Design review of the part built by this model. Coordinates are the model's own, in mm. A direction names the side the tool comes from. Coordinates: 2 decimals unless noted, no trailing zeros. Loops run counter-clockwise (first coordinate to the right, second up) from the corner with the lowest first, then second, coordinate; pieces in that order, holes last. Notation, with made-up numbers: (7, 81) -> (25, 81) arc R18 cw to (25, 111) -> close; hole circle Ø1 at (42, -0.75). An arc over 180 degrees is marked (long way). Use a Markdown table: item, result. Add a question column.
Q1. Take a section at B-B on y = -57. Write out the cut boundary in (x, z), plus the area to 3 significant figures.
Q2. Take a section at D-D on z = 0. Write out the cut boundary in (x, y), plus the area to 3 significant figures.
Q3. Draft analysis for pull direction X (two halves, no side actions). For faces 5 (the face through (99.84, 7.5, 8.86)), 6 (the face through (-12.5, 7, 0)), 7 (the face through (100, 7, -12.5)), state which applies: pulls with the +X half, pulls with the -X half, needs draft (parallel to the pull), parting line crosses it, or undercut.
Q4. Take a section at C-C on x = 47. Write out the cut boundary in (y, z).
Q5. Clearance check with flat-ended pins moving along their axes: pin 1 Ø1 at (x, z) = (44.5, 1) entering from -Y; pin 2 Ø12.5 at (x, z) = (95, -5.5) entering from -Y. State where each tip first meets the part, or that it passes through.
Q6. Take a section at A-A on z = -8.25. Write out the cut boundary in (x, y).
Q7. For faces 1 (the face through (87.5, 7, 0)), 2 (the face through (0.16, 7.5, -8.86)), 3 (the face through (100, 6, 12.5)), 4 (the face through (95.381, -36.975, -1.915)), list the 3-axis set-ups (+Z, -Z, +X, -X, +Y, -Y) from which the entire face can be reached by the end or side of a thin tool; tool diameter is ignored.
Q8. For probe 1 along X at (y, z) = (-62.5, -0.5); probe 2 along X at (y, z) = (3, -9.25); probe 3 along Y at (x, z) = (0, -8.75), list the stretches that pass through material, from the lowest coordinate up.
from build123d import *

# Parameters (mm, degrees)
SKETCH2_R           = 5
SKETCH4_W           = 25
SKETCH4_H           = 25
BOSS_EXTRUDE1_DEPTH = 15
SKETCH7_R           = 7.5
CUT_EXTRUDE2_DEPTH  = 15
SKETCH15_W          = 25
SKETCH15_H          = 25
BOSS_EXTRUDE3_DEPTH = 15
SKETCH17_R          = 7.5
CUT_EXTRUDE3_DEPTH  = 15


with BuildPart() as part:
    # Sweep1: sweep along a path in Sketch1
    with BuildLine(Plane.XY) as sweep1_path:
        Line((0, 0), (0, -75))
        ThreePointArc((0, -75), (4.393398122, -85.60660133), (14.999999452, -89.999999452))
        Line((14.999999452, -89.999999452), (85, -89.999999452))
        ThreePointArc((85, -89.999999452), (95.606601718, -85.60660117), (100, -74.999999452))
        Line((100, -74.999999452), (100, 0))
    # Sketch2 → Sweep1 (sweep)
    with BuildSketch(Plane(origin=(0, 0, 0), x_dir=(1, 0, 0), z_dir=(0, 1, 0))):
        Circle(SKETCH2_R)
    sweep(path=sweep1_path.line)

    # Sketch4 → Boss-Extrude1 (add)
    with BuildSketch(Plane(origin=(0, 0, 0), x_dir=(1, 0, 0), z_dir=(0, 1, 0))):
        Rectangle(SKETCH4_W, SKETCH4_H)
    extrude(amount=BOSS_EXTRUDE1_DEPTH)

    # Sketch5 → Cut-Revolve1 (revolve, cut)
    with BuildSketch(Plane(origin=(0, 15, 0), x_dir=(1, 0, 0), z_dir=(0, 1, 0))):
        with BuildLine():
            Line((0, 8.5), (0, -11.5))
            ThreePointArc((0, -11.5), (10, -1.5), (0, 8.5))
        make_face()
    revolve(axis=Axis((0, 15, -8.5), (0, 0, 1)), mode=Mode.SUBTRACT)

    # Sketch7 → Cut-Extrude2 (cut)
    with BuildSketch(Plane(origin=(0, 0, -12.5), x_dir=(-1, 0, 0), z_dir=(0, 0, -1))):
        with Locations((0, 15)):
            Circle(SKETCH7_R)
    extrude(amount=-CUT_EXTRUDE2_DEPTH, mode=Mode.SUBTRACT)

    # Sketch15 → Boss-Extrude3 (add)
    with BuildSketch(Plane(origin=(0, 0, 0), x_dir=(1, 0, 0), z_dir=(0, 1, 0))):
        with Locations((100, 0)):
            Rectangle(SKETCH15_W, SKETCH15_H)
    extrude(amount=BOSS_EXTRUDE3_DEPTH)

    # Sketch16 → Cut-Revolve2 (revolve, cut)
    with BuildSketch(Plane(origin=(0, 15, 0), x_dir=(1, 0, 0), z_dir=(0, 1, 0))):
        with BuildLine():
            Line((100, 11.5), (100, -8.5))
            ThreePointArc((100, -8.5), (110, 1.5), (100, 11.5))
        make_face()
    revolve(axis=Axis((100, 15, -11.5), (0, 0, 1)), mode=Mode.SUBTRACT)

    # Sketch17 → Cut-Extrude3 (cut)
    with BuildSketch(Plane.XY.offset(12.5)):
        with Locations((100, 15)):
            Circle(SKETCH17_R)
    extrude(amount=-CUT_EXTRUDE3_DEPTH, mode=Mode.SUBTRACT)


solid = part.part
Answer list:
| question | item | result |
|---|---|---|
| 1 | outline | circle Ø10 at (0, 0); circle Ø10 at (100, 0) |
| 1 | area | 157 mm² |
| 2 | outline | (-12.5, 0) -> (-5, 0) -> (-5, -75) arc R20 ccw to (15, -95) -> (85, -95) arc R20 ccw to (105, -75) -> (105, 0) -> (112.5, 0) -> (112.5, 15) -> (109.89, 15) arc R9.89 cw to (90.11, 15) -> (87.5, 15) -> (87.5, 0) -> (95, 0) -> (95, -75) arc R10 cw to (85, -85) -> (15, -85) arc R10 cw to (5, -75) -> (5, 0) -> (12.5, 0) -> (12.5, 15) -> (9.89, 15) arc R9.89 cw to (-9.89, 15) -> (-12.5, 15) -> close |
| 2 | area | 3,110 mm² |
| 3 | face 5 | undercut |
| 3 | face 6 | pulls with the -X half |
| 3 | face 7 | needs draft |
| 4 | outline | circle Ø10 at (-90, 0) |
| 5 | pin 1 | y = -94.97 |
| 5 | pin 2 | y = -94.09 |
| 6 | outline | (-12.5, 0) -> (12.5, 0) -> (12.5, 15) -> (7.5, 15) arc R7.5 cw to (-7.5, 15) -> (-12.5, 15) -> close; (87.5, 0) -> (112.5, 0) -> (112.5, 15) -> (107.38, 15) arc R7.38 cw to (92.62, 15) -> (87.5, 15) -> close |
| 7 | face 1 | +Z, -Z, +Y |
| 7 | face 2 | -Z, +Y |
| 7 | face 3 | +Z, +X, -X, +Y, -Y |
| 7 | face 4 | none |
| 8 | probe 1 | -4.97 to 4.97, 95.03 to 104.97 |
| 8 | probe 2 | -12.5 to 12.5, 87.5 to 112.5 |
| 8 | probe 3 | 0 to 7.5 |
